Autodesk Inventor part; units mm, degrees
ref_plane "YZ Plane" through (0, 0, 0) normal (1, 0, 0) x (0, 1, 0)
ref_plane "XZ Plane" through (0, 0, 0) normal (0, 1, 0) x (-1, 0, 0)
ref_plane "XY Plane" through (0, 0, 0) normal (0, 0, 1) x (1, 0, 0)
sketch "Sketch1" plane through (0, 0, 0) normal (0, 0, 1) x (1, 0, 0)
  line L0 (0, 0) -> (-23, 0)
  line L1 (-23, 0) -> (-23, 11)
  line L2 (-23, 11) -> (0, 11)
  line L3 (0, 11) -> (0, 0)
  line L4 (-17.8694, 8.961) -> (2.181, 8.961) construction
  line L5 (2.181, 8.961) -> (2.181, 1.8992) construction
  line L6 (2.181, 1.8992) -> (-17.8694, 1.8992) construction
  line L7 (-17.8694, 1.8992) -> (-17.8694, 8.961) construction
  line L8 (-16.745, 8.867) -> (-16.7294, 8.7729)
  line L9 (-16.7294, 8.7729) -> (-16.7294, 3.2097)
  line L10 (-16.7294, 3.2097) -> (-15.891, 3.2097)
  spline S0 degree 2 poles (-15.891, 3.2097) (-15.793, 3.1744) (-15.7773, 3.0647) knots 0 0 0 1 1 1
  spline S1 degree 2 poles (-15.7773, 3.0647) (-15.7773, 2.9707) (-15.8518, 2.861) (-15.9693, 2.861) knots 0 0 0 1 2 2 2
  line L11 (-15.9693, 2.861) -> (-17.9204, 2.861)
  spline S2 degree 2 poles (-17.9204, 2.861) (-18.0222, 2.8923) (-18.0379, 3.002) knots 0 0 0 1 1 1
  spline S3 degree 2 poles (-18.0379, 3.002) (-18.0379, 3.1) (-17.9478, 3.2097) (-17.7872, 3.2097) knots 0 0 0 1 2 2 2
  line L12 (-17.7872, 3.2097) -> (-17.078, 3.2097)
  line L13 (-17.078, 3.2097) -> (-17.078, 8.3577)
  line L14 (-17.078, 8.3577) -> (-17.7832, 7.672)
  spline S4 degree 2 poles (-17.7832, 7.672) (-17.8303, 7.6564) (-17.8655, 7.6564) knots 0 0 0 1 1 1
  spline S5 degree 2 poles (-17.8655, 7.6564) (-17.94, 7.6564) (-18.0379, 7.7465) (-18.0379, 7.8366) knots 0 0 0 1 2 2 2
  line L15 (-18.0379, 7.8366) -> (-18.0222, 7.911)
  line L16 (-18.0222, 7.911) -> (-16.9958, 8.9414)
  spline S6 degree 2 poles (-16.9958, 8.9414) (-16.9605, 8.9649) (-16.9017, 8.9649) knots 0 0 0 1 1 1
  spline S7 degree 2 poles (-16.9017, 8.9649) (-16.8861, 8.9649) (-16.7725, 8.914) (-16.745, 8.867) knots 0 0 0 1 2 2 2
  line L17 (-11.0368, 8.914) -> (-10.0339, 7.9032)
  line L18 (-10.0339, 7.9032) -> (-10.0182, 7.8288)
  line L19 (-10.0182, 7.8288) -> (-10.0182, 6.8258)
  line L20 (-10.0182, 6.8258) -> (-10.0339, 6.767)
  line L21 (-10.0339, 6.767) -> (-11.0642, 5.7562)
  line L22 (-11.0642, 5.7562) -> (-11.1387, 5.7327)
  line L23 (-11.1387, 5.7327) -> (-12.9918, 5.7327)
  line L24 (-12.9918, 5.7327) -> (-13.8537, 4.8826)
  line L25 (-13.8537, 4.8826) -> (-13.8537, 3.2097)
  line L26 (-13.8537, 3.2097) -> (-10.1514, 3.2097)
  spline S8 degree 2 poles (-10.1514, 3.2097) (-10.0182, 3.194) (-10.0182, 3.0373) knots 0 0 0 1 1 1
  spline S9 degree 2 poles (-10.0182, 3.0373) (-10.0182, 2.9589) (-10.0848, 2.861) (-10.2023, 2.861) knots 0 0 0 1 2 2 2
  line L27 (-10.2023, 2.861) -> (-14.0927, 2.861)
  spline S10 degree 2 poles (-14.0927, 2.861) (-14.1789, 2.8923) (-14.2024, 2.9668) knots 0 0 0 1 1 1
  line L28 (-14.2024, 2.9668) -> (-14.2024, 3.1352)
  line L29 (-14.2024, 3.1352) -> (-14.2024, 5.055)
  line L30 (-14.2024, 5.055) -> (-13.172, 6.0658)
  line L31 (-13.172, 6.0658) -> (-13.1211, 6.0814)
  line L32 (-13.1211, 6.0814) -> (-11.2327, 6.0814)
  line L33 (-11.2327, 6.0814) -> (-10.3669, 6.9433)
  line L34 (-10.3669, 6.9433) -> (-10.3669, 7.7543)
  line L35 (-10.3669, 7.7543) -> (-11.2209, 8.6162)
  line L36 (-11.2209, 8.6162) -> (-12.9996, 8.6162)
  line L37 (-12.9996, 8.6162) -> (-13.9438, 7.672)
  spline S11 degree 2 poles (-13.9438, 7.672) (-13.9947, 7.6564) (-14.03, 7.6564) knots 0 0 0 1 1 1
  spline S12 degree 2 poles (-14.03, 7.6564) (-14.1044, 7.6564) (-14.2024, 7.7465) (-14.2024, 7.8366) knots 0 0 0 1 2 2 2
  line L38 (-14.2024, 7.8366) -> (-14.1867, 7.911)
  line L39 (-14.1867, 7.911) -> (-13.1681, 8.9336)
  line L40 (-13.1681, 8.9336) -> (-13.1015, 8.9649)
  line L41 (-13.1015, 8.9649) -> (-11.0956, 8.9571)
  line L42 (-11.0956, 8.9571) -> (-11.0368, 8.914)
  spline S13 degree 2 poles (-8.1494, 4.1147) (-8.0985, 4.0716) (-8.0985, 3.9149) knots 0 0 0 1 1 1
  line L43 (-8.0985, 3.9149) -> (-8.0985, 2.9942)
  spline S14 degree 2 poles (-8.0985, 2.9942) (-8.1063, 2.9276) (-8.1886, 2.8767) knots 0 0 0 1 1 1
  spline S15 degree 2 poles (-8.1886, 2.8767) (-8.216, 2.861) (-8.2708, 2.861) knots 0 0 0 1 1 1
  spline S16 degree 2 poles (-8.2708, 2.861) (-8.357, 2.861) (-8.4471, 2.9354) (-8.4471, 3.0451) knots 0 0 0 1 2 2 2
  line L44 (-8.4471, 3.0451) -> (-8.4471, 4.0442)
  spline S17 degree 2 poles (-8.4471, 4.0442) (-8.4158, 4.1617) (-8.2983, 4.1617) knots 0 0 0 1 1 1
  spline S18 degree 2 poles (-8.2983, 4.1617) (-8.1964, 4.1617) (-8.1494, 4.1147) knots 0 0 0 1 1 1
  line L45 (-4.3296, 8.9336) -> (-3.3188, 7.9149)
  line L46 (-3.3188, 7.9149) -> (-3.3031, 7.864)
  line L47 (-3.3031, 7.864) -> (-3.3266, 3.8875)
  line L48 (-3.3266, 3.8875) -> (-4.357, 2.8688)
  line L49 (-4.357, 2.8688) -> (-4.4118, 2.861)
  line L50 (-4.4118, 2.861) -> (-5.4579, 2.861)
  line L51 (-5.4579, 2.861) -> (-5.5088, 2.8923)
  line L52 (-5.5088, 2.8923) -> (-6.5196, 3.911)
  line L53 (-6.5196, 3.911) -> (-6.5274, 3.9972)
  line L54 (-6.5274, 3.9972) -> (-6.4961, 7.9463)
  line L55 (-6.4961, 7.9463) -> (-5.4735, 8.9492)
  line L56 (-5.4735, 8.9492) -> (-5.4265, 8.9649)
  line L57 (-5.4265, 8.9649) -> (-4.3962, 8.9571)
  line L58 (-4.3962, 8.9571) -> (-4.3296, 8.9336)
  line L59 (-3.6518, 7.7543) -> (-4.5059, 8.6084)
  line L60 (-4.5059, 8.6084) -> (-5.3247, 8.6084)
  line L61 (-5.3247, 8.6084) -> (-6.1787, 7.7543)
  line L62 (-6.1787, 7.7543) -> (-6.1787, 4.0638)
  line L63 (-6.1787, 4.0638) -> (-5.3247, 3.2097)
  line L64 (-5.3247, 3.2097) -> (-4.5059, 3.2097)
  line L65 (-4.5059, 3.2097) -> (-3.6518, 4.0716)
  line L66 (-3.6518, 4.0716) -> (-3.6518, 7.7543)
  dimension "d0" = 23
  dimension "d1" = 11
extrude "Extrusion1" add sketch "Sketch1" against normal blind 10 contours L0 L1 L2 L3 | L8 L9 L10 S0 S1 L11 S2 S3 L12 L13 L14 S4 S5 L15 L16 S6 S7 | L17 L18 L19 L20 L21 L22 L23 L24 L25 L26 S8 S9 L27 S10 L28 L29 L30 L31 L32 L33 L34 L35 L36 L37 S11 S12 L38 L39 L40 L41 L42 | S13 L43 S14 S15 S16 L44 S17 S18 | L45 L46 L47 L48 L49 L50 L51 L52 L53 L54 L55 L56 L57 L58 | L66 L65 L64 L63 L62 L61 L60 L59
extrude "Extrusion2" add sketch "Sketch1" along normal blind 1 contours L8 L9 L10 S0 S1 L11 S2 S3 L12 L13 L14 S4 S5 L15 L16 S6 S7 | L17 L18 L19 L20 L21 L22 L23 L24 L25 L26 S8 S9 L27 S10 L28 L29 L30 L31 L32 L33 L34 L35 L36 L37 S11 S12 L38 L39 L40 L41 L42 | S13 L43 S14 S15 S16 L44 S17 S18 | L45 L46 L47 L48 L49 L50 L51 L52 L53 L54 L55 L56 L57 L58
properties part number "VolteMeter"
For this review, take the finished solid that the model builds, in its own axes (mm). A direction names the side the tool comes from. Round coordinates to 2 decimals unless told otherwise and drop trailing zeros. Write each loop counter-clockwise with the first axis right and the second up, starting at its lowest first coordinate (ties: lowest second). Pieces come first, ordered by that corner, then holes. Notation, with made-up numbers: (51.25, 61) -> (108.25, 61) arc R25 ccw to (108.25, 83) -> close; hole circle Ø3 at (15, -39.75). An arc over 180 degrees is marked (long way). Use CSV: the item, a comma, the result in double quotes.
(1) For faces 5 (the face through (-12.2, 6.081, 0.5)), 6 (the face through (-5.99, 8.44, 0.49)), 7 (the face through (-6.36, 5.93, 1)), 8 (the face through (-3.83, 3.39, 0.49)), 9 (the face through (-8.447, 3.5, 0.5)), list the 3-axis set-ups (+Z, -Z, +X, -X, +Y, -Y) from which the entire face can be reached by the end or side of a thin tool; tool diameter is ignored.
Computed values:
face 5,"+Z"
face 6,"+Z, +Y"
face 7,"+Z, +X, -X, +Y, -Y"
face 8,"+Z, +X, -Y"
face 9,"+Z, +Y, -Y"
(2) Consider section B-B, the plane x = -12.5. Give the boundary of the cut face in (y, z), plus the area to 3 significant figures.
Computed values:
outline,"(0, -10) -> (11, -10) -> (11, 0) -> (8.96, 0) -> (8.96, 1) -> (8.62, 1) -> (8.62, 0) -> (6.08, 0) -> (6.08, 1) -> (5.73, 1) -> (5.73, 0) -> (3.21, 0) -> (3.21, 1) -> (2.86, 1) -> (2.86, 0) -> (0, 0) -> close"
area,"111 mm²"
(3) Consider section A-A, the plane y = 5.5. Give the boundary of the cut face in (x, z).
Computed values:
outline,"(-23, -10) -> (0, -10) -> (0, 0) -> (-3.32, 0) -> (-3.32, 1) -> (-3.65, 1) -> (-3.65, 0) -> (-6.18, 0) -> (-6.18, 1) -> (-6.52, 1) -> (-6.52, 0) -> (-13.23, 0) -> (-13.23, 1) -> (-13.75, 1) -> (-13.75, 0) -> (-16.73, 0) -> (-16.73, 1) -> (-17.08, 1) -> (-17.08, 0) -> (-23, 0) -> close"
(4) Clearance check with flat-ended pins moving along their axes: P1, Ø0.7, axis at x = -5, z = 0.5, coming from the -Y side; P2, Ø0.8, axis at y = 7, z = 0.5, coming from the +X side; P3, Ø0.8, axis at x = -12, z = 0.5, coming from the +Y side. State where each tip first meets the part, or that it passes through.
Computed values:
P1,"y = 2.86"
P2,"x = -3.31"
P3,"y = 8.96"
(5) Draft analysis for pull direction X (two halves, no side actions). For faces 1 (the face through (-5, 6, 0)), 2 (the face through (-3.8, 8.4, 0.5)), 3 (the face through (-23, 5, -5)), 4 (the face through (-16.9, 5.9, 1)), state which applies: +X half, -X half, draft (parallel to the pull), parting line (faces both ways), or undercut.
Computed values:
face 1,"undercut"
face 2,"+X half"
face 3,"-X half"
face 4,"draft"
(6) To check wall thickness, follow L1, parallel to Z at x = -2.5, y = 10.25. State the ranges of the line that lie inside material, in increasing order. Write a range as [from, to].
Computed values:
L1,"[-10, 0]"
(7) Consider section C-C, the plane y = 1.75. Give the boundary of the cut face in (x, z).
Computed values:
outline,"(-23, -10) -> (0, -10) -> (0, 0) -> (-23, 0) -> close"
(8) Consider section D-D, the plane x = -4.75. Give the boundary of the cut face in (y, z).
Computed values:
outline,"(0, -10) -> (11, -10) -> (11, 0) -> (8.96, 0) -> (8.96, 1) -> (8.61, 1) -> (8.61, 0) -> (3.21, 0) -> (3.21, 1) -> (2.86, 1) -> (2.86, 0) -> (0, 0) -> close"
